Build history of the part. All positions in model axes, mm. Face numbers are marked on the shaded views. A direction names the side the tool comes from. Give positions to 0.01 mm unless a question says otherwise; leave off trailing zeros. Write each loop counter-clockwise with the first axis right and the second up, starting at its lowest first coordinate (ties: lowest second). Pieces come first, ordered by that corner, then holes. Notation, with made-up numbers: M 29,49.5 L 37,49.5 A15 cw 37,56.5 Z; hole C 40,0.25 d9. An arc over 180 degrees is marked long. Return JSON: item names as keys, results as strings. Group by question number.
Q1. Wall check: probe 1 along X at (y, z) = (-8.25, 2.5); probe 2 along Y at (x, z) = (-8.5, 0.5); probe 3 along Z at (x, y) = (11, 11). Give the ranges that are in metal, low to high.
Q2. Flat gauge pins, fed straight in: pin 1 Ø1.5 at (x, z) = (10, 1.5) entering from -Y; pin 2 Ø2 at (y, z) = (-16.5, 1.5) entering from -X; pin 3 Ø3 at (x, y) = (-6.5, -8.5) entering from -Z; pin 4 Ø1.5 at (x, z) = (-25, 1.5) entering from +Y. Where does each tip first touch, or does it go through?
Q3. Band-saw the part on B-B, the plane x = -10.5. Give the cut face in (y, z), then the cut area to 3 significant figures.
Q4. Band-saw the part on A-A, the plane y = 1.5. Give the cut face in (x, z), then the cut area to 3 significant figures.
Q5. Pull direction X, two halves, no side cores. Call the marked faces 4, 5 and 6: +X half, -X half, draft (parallel to the pull), parting line (faces both ways), or undercut.
Q6. Band-saw the part on C-C, the plane y = 13.5. Give the cut face in (x, z), then the cut area to 3 significant figures.
Q7. Band-saw the part on D-D, the plane y = -11. Give the cut face in (x, z), then the cut area to 3 significant figures.
Q8. Tool access for the marked faces 1, 2 and 3: list every direction of +Z, -Z, +X, -X, +Y, -Y with a clear straight run to the whole face (end or side of a thin tool).
Autodesk Inventor part; units mm, degrees
ref_plane "YZ Plane" through (0, 0, 0) normal (1, 0, 0) x (0, 1, 0)
ref_plane "XZ Plane" through (0, 0, 0) normal (0, 1, 0) x (-1, 0, 0)
ref_plane "XY Plane" through (0, 0, 0) normal (0, 0, 1) x (1, 0, 0)
sketch "Sketch1" plane through (0, 0, 0) normal (0, 0, 1) x (1, 0, 0)
  line L0 (-55, -19.25) -> (14, -19.25)
  line L1 (14, -19.25) -> (14, 19.25)
  line L2 (14, 19.25) -> (-55, 19.25)
  line L3 (-55, 19.25) -> (-55, -19.25)
  line L4 (-55, -19.25) -> (14, 19.25) construction
  line L5 (14, -19.25) -> (-55, 19.25) construction
  line L6 (14, -6.05) -> (9, -6.05)
  line L7 (9, -6.05) -> (9, 6.05)
  line L8 (9, 6.05) -> (14, 6.05)
  line L9 (14, 0) -> (-55, 0)
  line L10 (-4, 14.25) -> (-37, 14.25)
  arc A0 (9, 6.05) -> (9, 3.05) centre (9, 4.55) ccw
  arc A1 (9, -3.05) -> (9, -6.05) centre (9, -4.55) ccw
  line L11 (-4, -14.25) -> (-37, -14.25)
  line L12 (-20.5, -19.25) -> (-20.5, 19.25) construction
  line L13 (-55, -6.05) -> (-50, -6.05)
  line L14 (-50, -6.05) -> (-50, 6.05)
  line L15 (-50, 6.05) -> (-55, 6.05)
  arc A2 (-50, 3.05) -> (-50, 6.05) centre (-50, 4.55) ccw
  arc A3 (-50, -6.05) -> (-50, -3.05) centre (-50, -4.55) ccw
  line L16 (5, -10.25) -> (5, 10.25)
  line L17 (5, 10.25) -> (-46, 10.25)
  line L18 (5, -10.25) -> (-46, -10.25)
  line L19 (-46, -10.25) -> (-46, 10.25)
  line L20 (-55, -14.25) -> (-46, -14.25)
  line L21 (-46, -14.25) -> (-46, -19.25)
  line L22 (-37, -19.25) -> (-37, -14.25)
  arc A4 (-46, -14.25) -> (-49, -14.25) centre (-47.5, -14.25) ccw
  arc A5 (-34, -14.25) -> (-37, -14.25) centre (-35.5, -14.25) ccw
  line L23 (-55, 14.25) -> (-46, 14.25)
  line L24 (-46, 14.25) -> (-46, 19.25)
  line L25 (-37, 19.25) -> (-37, 14.25)
  arc A6 (-49, 14.25) -> (-46, 14.25) centre (-47.5, 14.25) ccw
  arc A7 (-37, 14.25) -> (-34, 14.25) centre (-35.5, 14.25) ccw
  line L26 (-52, 14.25) -> (-52, 8.25) construction
  line L27 (14, 6) -> (9, 6) construction
  line L28 (14, -6) -> (9, -6) construction
  line L29 (-4, 19.25) -> (-4, 14.25)
  line L30 (14, 14.25) -> (5, 14.25)
  line L31 (5, 14.25) -> (5, 19.25)
  line L32 (11, 14.25) -> (11, 8.25) construction
  arc A8 (5, 14.25) -> (8, 14.25) centre (6.5, 14.25) ccw
  arc A9 (-7, 14.25) -> (-4, 14.25) centre (-5.5, 14.25) ccw
  line L33 (-4, -19.25) -> (-4, -14.25)
  line L34 (14, -14.25) -> (5, -14.25)
  line L35 (5, -14.25) -> (5, -19.25)
  arc A10 (8, -14.25) -> (5, -14.25) centre (6.5, -14.25) ccw
  arc A11 (-4, -14.25) -> (-7, -14.25) centre (-5.5, -14.25) ccw
  point P0 (0, 0)
  point P1 (-20.5, 0)
  point P2 (-55, 6.05)
  point P3 (-55, -6.05)
  point P4 (-37, 19.25)
  point P5 (-55, 14.25)
  point P6 (-34, 14.25)
  point P7 (5, 0)
  point P8 (9, 0)
  point P9 (-50, 0)
  point P10 (-46, 0)
  dimension "d0" = 38.5
  dimension "d2" = 12.1
  dimension "d3" = 14
  dimension "d4" = 5
  dimension "d12" = 1.5
  dimension "d27" = 69
  dimension "d36" = 2.5
  dimension "d40" = 9
  dimension "d42" = 6
  dimension "d51" = 2.5
  dimension "d55" = 12
  dimension "d56" = 0.05
  dimension "d57" = 5
  dimension "d58" = 9
  dimension "d59" = 6
  dimension "d70" = 9
extrude "Extrusion1" add sketch "Sketch1" along normal blind 5 contours L3 L23 A6 L24 L2 L25 A7 L10 A9 L29 L31 A8 L30 L1 L8 A0 L7 L9 L16 L17 L19 L14 A2 L15
fillet "Fillet1" radius 2 2 edges at (5, 10.25, 2.5) (-46, 10.25, 2.5)
sketch "Sketch5" plane through (-34, 14.25, 0) normal (0, 1, 0) x (1, 0, 0)
  line L0 (45, 0) -> (45, -5)
  line L1 (43, -5) -> (48, -5)
  line L2 (-18, 0) -> (-18, -5)
  line L3 (-15, -5) -> (-21, -5)
  point P0 (34, 0)
  point P1 (45, -2.5)
  point P2 (-18, -2.5)
hole "Hole1" at (11, 14.25, 2.5) at (-52, 14.25, 2.5) direction (0, -1, 0) diameter 2.459 depth 8.8
chamfer "Chamfer1" distance 0.5 angle 45 6 edges at (14, 6.05, 2.5) (5, 19.25, 2.5) (-4, 19.25, 2.5) (-37, 19.25, 2.5) (-46, 19.25, 2.5) (-55, 6.05, 2.5)
mirror "Mirror1" about plane through (0, 0, 0) normal (0, 1, 0)
equation "\"d42\" = d6"
properties part number "LegBaseBraceFrame" material "Acetal Resin, Black"
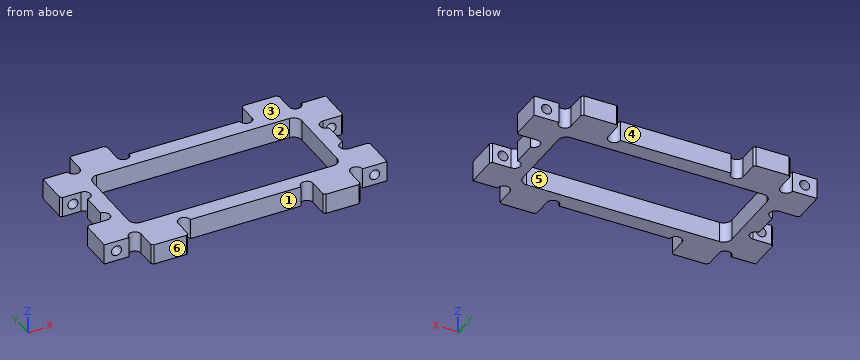
From the geometry:
{
 "1": {"probe 1": "x = -55 to -53.23, -50.77 to -46, 5 to 9.77, 12.23 to 14", "probe 2": "y = -14.25 to -10.25, 10.25 to 14.25", "probe 3": "z = 0 to 1.27, 3.73 to 5"},
 "2": {"pin 1": "stops at y = -14.25", "pin 2": "stops at x = -46", "pin 3": "passes through", "pin 4": "stops at y = 14.25"},
 "3": {"outline": "M -14.25,0 L -10.25,0 L -10.25,5 L -14.25,5 Z; M 10.25,0 L 14.25,0 L 14.25,5 L 10.25,5 Z", "area": "40.0 mm^2"},
 "4": {"outline": "M -50,0 L -46,0 L -46,5 L -50,5 Z; M 5,0 L 9,0 L 9,5 L 5,5 Z", "area": "40.0 mm^2"},
 "5": {"face 4": "undercut", "face 5": "undercut", "face 6": "draft"},
 "6": {"outline": "M -55,0 L -48.8,0 L -48.8,5 L -55,5 Z; M -46.2,0 L -36.8,0 L -36.8,5 L -46.2,5 Z; M -34.2,0 L -6.8,0 L -6.8,5 L -34.2,5 Z; M -4.2,0 L 5.2,0 L 5.2,5 L -4.2,5 Z; M 7.8,0 L 14,0 L 14,5 L 7.8,5 Z; hole C -52,2.5 d2.46; hole C 11,2.5 d2.46", "area": "284 mm^2"},
 "7": {"outline": "M -55,0 L 14,0 L 14,5 L -55,5 Z; hole C -52,2.5 d2.46; hole C 11,2.5 d2.46", "area": "336 mm^2"},
 "8": {"face 1": "+Z, -Z, -Y", "face 2": "+Z, -Z", "face 3": "+Z, +X, -X, +Y, -Y"}
}
